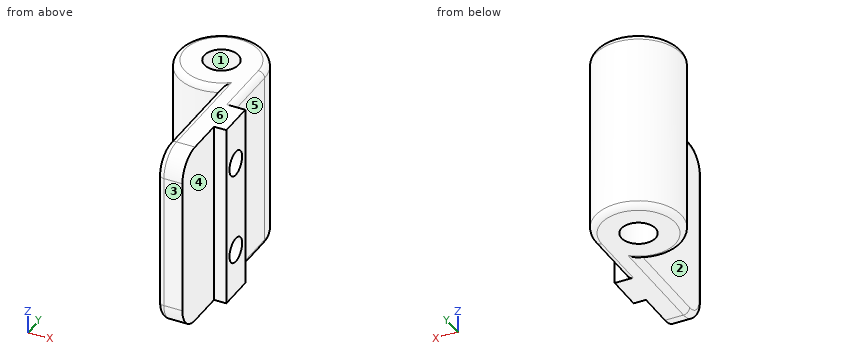
from build123d import *

# Parameters (mm, degrees)
SKETCH_R     = 2.777235
PAD_DEPTH    = 30
SKETCH001_W  = 6
SKETCH001_H  = 30
PAD001_DEPTH = 2
SKETCH002_R  = 2
POCKET_DEPTH = 6
FILLET_R     = 4
FILLET001_R  = 4
FILLET002_R  = 1
FILLET003_R  = 1
FILLET004_R  = 1


with BuildPart() as part:
    # Sketch → Pad (new body)
    with BuildSketch(Plane.XY):
        with BuildLine():
            Line((14, 0), (14, -26))
            Line((14, -26), (10, -26))
            Line((10, -26), (10, -6.324555))
            ThreePointArc((14, 0), (1.08392, 3.741657), (10, -6.324555))
        make_face()
        with Locations((7, 0)):
            Circle(SKETCH_R, mode=Mode.SUBTRACT)
    extrude(amount=PAD_DEPTH)

    # Sketch001 → Pad001 (new body)
    with BuildSketch(Plane.YZ.offset(14)):
        with Locations((-13, 15)):
            Rectangle(SKETCH001_W, SKETCH001_H)
    extrude(amount=PAD001_DEPTH)

    # Sketch002 → Pocket (cut)
    with BuildSketch(Plane.YZ.offset(16)):
        with Locations((-13, 22.5)):
            Circle(SKETCH002_R)
        with Locations((-13, 7.5)):
            Circle(SKETCH002_R)
    extrude(amount=-POCKET_DEPTH, mode=Mode.SUBTRACT)

    # Fillet
    fillet_edges = [part.edges().sort_by_distance(p)[0] for p in [
        (12, -26, 0),
    ]]
    fillet(fillet_edges, radius=FILLET_R)

    # Fillet001
    fillet001_edges = [part.edges().sort_by_distance(p)[0] for p in [
        (12, -26, 30),
    ]]
    fillet(fillet001_edges, radius=FILLET001_R)

    # Fillet002
    fillet002_edges = [part.edges().sort_by_distance(p)[0] for p in [
        (10, -26, 15),
    ]]
    fillet(fillet002_edges, radius=FILLET002_R)

    # Fillet003
    fillet003_edges = [part.edges().sort_by_distance(p)[0] for p in [
        (1.08392, 3.741657, 30),
    ]]
    fillet(fillet003_edges, radius=FILLET003_R)

    # Fillet004
    fillet004_edges = [part.edges().sort_by_distance(p)[0] for p in [
        (1.08392, 3.741657, 0),
    ]]
    fillet(fillet004_edges, radius=FILLET004_R)


solid = part.part
Geometry: final body of the model. Coordinates: model frame, mm. Face numbers are marked on the shaded views. A direction names the side the tool comes from. Coordinates: 2 decimals unless noted, no trailing zeros. Loops run counter-clockwise (first coordinate to the right, second up) from the corner with the lowest first, then second, coordinate; pieces in that order, holes last. Notation, with made-up numbers: (89.5, 24) - (96.5, 24) arc R19 ccw to (96.5, 32) - close; hole circle Ø5 at (10.25, 14.5). An arc over 180 degrees is marked (long way). Put each result on its own line as item: value. Start each with the question number.
Q1. Pin query (flat end, axial travel): pin 1 Ø0.6 at (x, z) = (14.5, 15) entering from -Y; pin 2 Ø8 at (y, z) = (-3, 15) entering from +X; pin 3 Ø1 at (x, z) = (4, 19.5) entering from +Y. Return the tip coordinate at first contact, or that it passes through.
Q2. Set-up query: the marked faces 4, 5 and 6. Return all of +Z, -Z, +X, -X, +Y, -Y with unobstructed straight access to the full face (end or side cutting, diameter ignored); none if empty.
Q3. Cut plane B-B, the plane z = 23. Return loops of the section in (x, y).
Q4. Line query: line 1 (Z direction, x = 11.5, y = -13); line 2 (Y direction, x = 7, z = 26); line 3 (X direction, y = -18, z = 17). Output: solid intervals per line, ascending.
Q5. Cut plane C-C, the plane y = -16.5. Return loops of the section in (x, z).
Q6. Pull-direction query (Y, two-part tool) for the marked faces 1, 2 and 3; classes: released by +Y, released by -Y, zero draft, split by the parting line, or undercut.
Q7. Cut plane A-A, the plane z = 5. Return loops of the section in (x, y).
Filled sheet:
1. pin 1: y = -16
1. pin 2: x = 14
1. pin 3: y = 6.54
2. face 4: +Z, -Z, +X, -Y
2. face 5: +Z, -Z, +X, +Y
2. face 6: +Z, +X, -X, +Y, -Y
3. outline: (10, -25) arc R1 ccw to (11, -26) - (14, -26) - (14, -16) - (16, -16) - (16, -14.94) - (10, -14.94) - close; (10, -11.06) - (16, -11.06) - (16, -10) - (14, -10) - (14, 0) arc R7 ccw (long way) to (10, -6.32) - close; hole circle Ø5.55 at (7, 0)
4. line 1: 0 to 5.5, 9.5 to 20.5, 24.5 to 30
4. line 2: -7 to -2.78, 2.78 to 7
4. line 3: 10 to 14
5. outline: (10, 1) arc R1 ccw to (11, 0) - (14, 0) - (14, 30) - (11, 30) arc R1 ccw to (10, 29) - close
6. face 1: undercut
6. face 2: zero draft
6. face 3: released by -Y
7. outline: (10, -25) arc R1 ccw to (11, -26) - (14, -26) - (14, -16) - (16, -16) - (16, -10) - (14, -10) - (14, 0) arc R7 ccw (long way) to (10, -6.32) - close; hole circle Ø5.55 at (7, 0)
